Study the drawing (mm; zero at the part's minimum x, y, z) and answer. A direction names the side the tool comes from. Give positions to 0.01 mm unless a question says otherwise; leave off trailing zeros. Write each loop counter-clockwise with the first axis right and the second up, starting at its lowest first coordinate (ties: lowest second). Pieces come first, ordered by that corner, then holes.
1) Given pin 1 Ø6 at (x, y) = (25.5, 3) entering from -Z; pin 2 Ø10 at (y, z) = (18.5, 40) entering from -X; pin 3 Ø4 at (x, y) = (55, 11.5) entering from -Z, each flat-ended and moving along its own axis, determine where each tip first touches the part or whether it passes through.
2) Determine the mould class of the marked faces 4, 5 and 6 for opening direction X: pulls with the +X half, pulls with the -X half, needs draft (parallel to the pull), parting line crosses it, or undercut.
3) Find section C-C (x = 42). Determine the outline of the cut face in (y, z).
4) A tool of negligible diameter and unlimited length cuts with its end or side. For the marked faces 1, 2 and 3, from which of +Z, -Z, +X, -X, +Y, -Y can it reach the whole face along a straight path? Write none if from no direction.
5) Find section B-B (y = 5). Determine the outline of the cut face in (x, z).
6) Straight lines are drawn through the part: probe 1 along X at (y, z) = (1.25, 68); probe 2 along X at (y, z) = (8.5, 54); probe 3 along X at (y, z) = (1.5, 7.5). For each, find the intervals that lie inside material, in ascending order.
7) Find section D-D (z = 58). Determine the outline of the cut face in (x, y).
8) Find section A-A (z = 67). Determine the outline of the cut face in (x, y), plus the area to 3 significant figures.
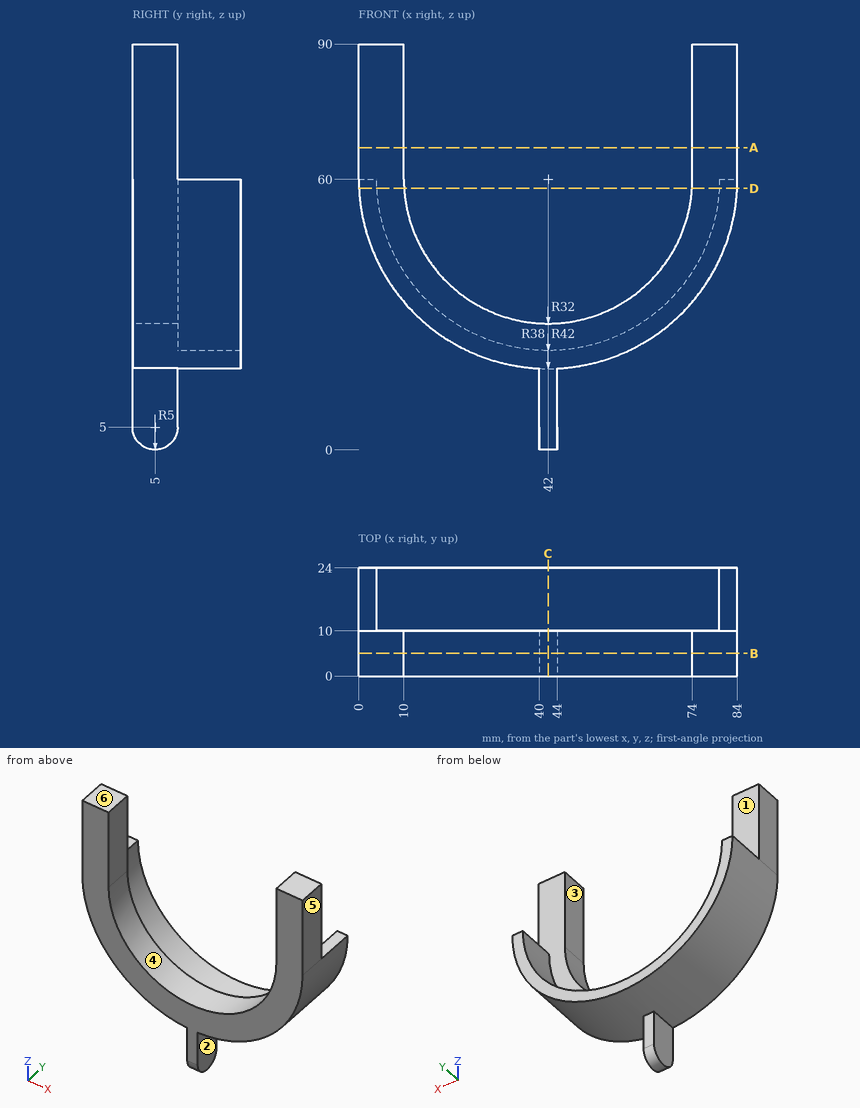
Results:
1. pin 1: stops at z = 20.23
1. pin 2: stops at x = 2.77
1. pin 3: stops at z = 19.47
2. face 4: undercut
2. face 5: pulls with the +X half
2. face 6: needs draft
3. outline: (0, 5) arc R5 ccw to (10, 5) - (10, 18) - (24, 18) - (24, 22) - (10, 22) - (10, 28) - (0, 28) - close
4. face 1: +Z, +Y
4. face 2: -Z, +X, +Y, -Y
4. face 3: +Z, +Y, -Y
5. outline: (0, 60) arc R42 ccw to (40, 18.05) - (40, 0) - (44, 0) - (44, 18.05) arc R42 ccw to (84, 60) - (84, 90) - (74, 90) - (74, 60) arc R32 cw to (10, 60) - (10, 90) - (0, 90) - close
6. probe 1: x = 0 to 10, 74 to 84
6. probe 2: x = 0.43 to 10.57, 73.43 to 83.57
6. probe 3: x = 40 to 44
7. outline: (0.05, 0) - (10.06, 0) - (10.06, 10) - (4.05, 10) - (4.05, 24) - (0.05, 24) - close; (73.94, 0) - (83.95, 0) - (83.95, 24) - (79.95, 24) - (79.95, 10) - (73.94, 10) - close
8. outline: (0, 0) - (10, 0) - (10, 10) - (0, 10) - close; (74, 0) - (84, 0) - (84, 10) - (74, 10) - close
8. area: 200 mm2
